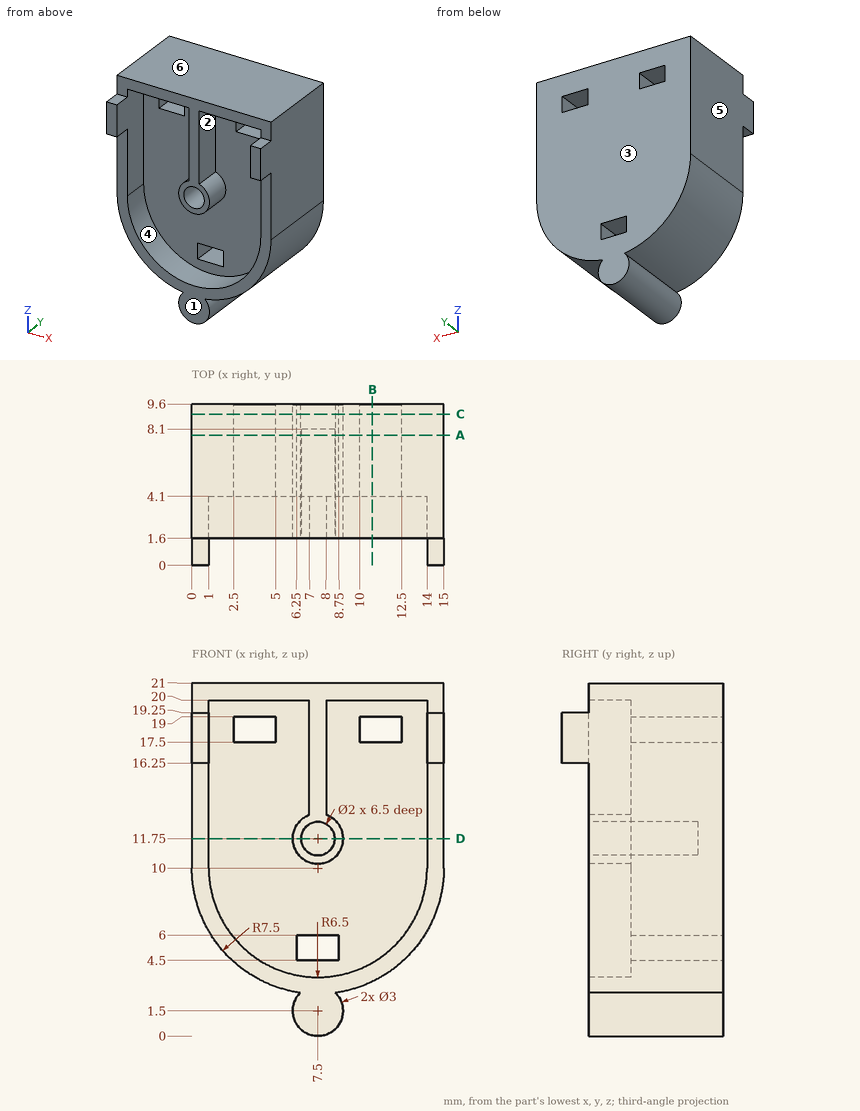
Answer from the drawing. Dimensions are ordinates in mm from the lowest x, y and z of the part. A direction names the side the tool comes from. Round coordinates to 2 decimals unless told otherwise and drop trailing zeros. Loops run counter-clockwise (first coordinate to the right, second up) from the corner with the lowest first, then second, coordinate; pieces in that order, holes last.
(1) The mould has two halves that part along Z. Classify the marked faces 4, 5 and 6: pulls with the +Z half, pulls with the -Z half, needs draft (parallel to the pull), parting line crosses it, or undercut.
Computed values:
face 4: undercut
face 5: needs draft
face 6: pulls with the +Z half
(2) For the marked faces 1, 2 and 3, determine the directions among +Z, -Z, +X, -X, +Y, -Y from which every point of the face is accessible in a straight line to the end or side of a thin tool.
Computed values:
face 1: -Z, +X, -X, -Y
face 2: -Y
face 3: +Z, -Z, +X, -X, +Y
(3) Find the intervals of material crossed by L1, parallel to X at y = 9.25, z = 18; L2, parallel to Z at x = 7.5, y = 6; L3, parallel to X at y = 2.75, z = 19.25, in increasing order.
Computed values:
L1: x = 0 to 2.5, 5 to 10, 12.5 to 15
L2: z = 0 to 4.5, 6 to 10.75, 12.75 to 21
L3: x = 0 to 1, 7 to 8, 14 to 15
(4) The part is cut by section C-C, the plane y = 9. Give the vertices of the cut face in (x, z), and give its area (3 significant figures).
Computed values:
outline: (0, 10) arc R7.5 ccw to (6.45, 2.57) arc R1.5 ccw (long way) to (8.55, 2.57) arc R7.5 ccw to (15, 10) - (15, 21) - (0, 21) - close; hole (2.5, 17.5) - (5, 17.5) - (5, 19) - (2.5, 19) - close; hole (6.25, 4.5) - (8.75, 4.5) - (8.75, 6) - (6.25, 6) - close; hole (10, 17.5) - (12.5, 17.5) - (12.5, 19) - (10, 19) - close
area: 248 mm2
(5) Each of these flat-tipped pins is pushed along its axis until it touches: P1, Ø2, axis at x = 3.5, z = 5.5, coming from the -Y side; P2, Ø0.6, axis at x = 8, z = 11.5, coming from the -Y side; P3, Ø0.8, axis at x = 0.5, y = 0.5, coming from the -Z side. Where does it stop, or does it pass through?
Computed values:
P1: stops at y = 1.6
P2: stops at y = 8.1
P3: stops at z = 16.25
(6) The part is cut by section D-D, the plane z = 11.75. Give the vertices of the cut face in (x, y).
Computed values:
outline: (0, 1.6) - (1, 1.6) - (1, 4.1) - (6, 4.1) - (6, 1.6) - (6.5, 1.6) - (6.5, 8.1) - (8.5, 8.1) - (8.5, 1.6) - (9, 1.6) - (9, 4.1) - (14, 4.1) - (14, 1.6) - (15, 1.6) - (15, 9.6) - (0, 9.6) - close
(7) The part is cut by section B-B, the plane x = 10.75. Give the vertices of the cut face in (y, z), and give its area (3 significant figures).
Computed values:
outline: (1.6, 3.24) - (9.6, 3.24) - (9.6, 17.5) - (4.1, 17.5) - (4.1, 4.37) - (1.6, 4.37) - close; (1.6, 20) - (4.1, 20) - (4.1, 19) - (9.6, 19) - (9.6, 21) - (1.6, 21) - close
area: 94.8 mm2
(8) The part is cut by section A-A, the plane y = 7.75. Give the vertices of the cut face in (x, z).
Computed values:
outline: (0, 10) arc R7.5 ccw to (6.45, 2.57) arc R1.5 ccw (long way) to (8.55, 2.57) arc R7.5 ccw to (15, 10) - (15, 21) - (0, 21) - close; hole (2.5, 17.5) - (5, 17.5) - (5, 19) - (2.5, 19) - close; hole (6.25, 4.5) - (8.75, 4.5) - (8.75, 6) - (6.25, 6) - close; hole circle Ø2 at (7.5, 11.75); hole (10, 17.5) - (12.5, 17.5) - (12.5, 19) - (10, 19) - close
